```python
from build123d import *

# Parameters (mm, degrees)
BOSS_EXTRUDE1_DEPTH         = 50
BOSS_EXTRUDE2_START         = -50
BOSS_EXTRUDE2_DEPTH         = 50
TAP_DRILL_FOR_M5X0_8_TAP1_D = 4.2
CUT_EXTRUDE1_REACH          = 69.195
SKETCH5_W                   = 63.468496122
SKETCH5_H                   = 5.35


with BuildPart() as part:
    # Sketch1 → Boss-Extrude1 (new body)
    with BuildSketch(Plane.XY):
        with BuildLine():
            Line((-31.734248061, 1), (-17.721808598, 1))
            ThreePointArc((-17.721808598, 1), (0, 17.75), (17.721808598, 1))
            Line((17.721808598, 1), (31.734248061, 1))
            ThreePointArc((31.734248061, 1), (0, 31.75), (-31.734248061, 1))
        make_face()
    extrude(amount=BOSS_EXTRUDE1_DEPTH)

    # Sketch4 → Boss-Extrude2 (add)
    with BuildSketch(Plane.XY.offset(50).offset(BOSS_EXTRUDE2_START)):
        with BuildLine():
            Line((31.734248061, 31.75), (0, 31.75))
            ThreePointArc((0, 31.75), (22.094258304, 22.801452805), (31.734248061, 1))
            Line((31.734248061, 1), (31.734248061, 31.75))
        make_face()
        with BuildLine():
            ThreePointArc((-31.734248061, 1), (-22.094258304, 22.801452805), (0, 31.75))
            Line((0, 31.75), (-31.734248061, 31.75))
            Line((-31.734248061, 31.75), (-31.734248061, 1))
        make_face()
    extrude(amount=BOSS_EXTRUDE2_DEPTH)

    # Tap Drill for M5x0.8 Tap1 (through all)
    with Locations(Plane(origin=(-24.72802833, 1, 40), x_dir=(0, 0, -1), z_dir=(0, -1, 0))):
        with Locations((0, 0), (30, 0), (0, 49.45605666), (30, 49.45605666)):
            Hole(TAP_DRILL_FOR_M5X0_8_TAP1_D / 2)

    # Sketch5 → Cut-Extrude1 (cut, up to next)
    with BuildSketch(Plane.XY.offset(50), mode=Mode.PRIVATE) as cut_extrude1_sk1:
        with Locations((0, 29.075)):
            Rectangle(SKETCH5_W, SKETCH5_H)
    cut_extrude1_tool1 = extrude(cut_extrude1_sk1.sketch, amount=-CUT_EXTRUDE1_REACH, mode=Mode.PRIVATE) & part.part
    add(cut_extrude1_tool1.solids().sort_by_distance((0, 29.075, 50))[0], mode=Mode.SUBTRACT)


solid = part.part
```
Here's how the part is built. I have some questions about the finished solid (model axes, mm). Coordinates: 2 decimals unless noted, no trailing zeros. Loops run counter-clockwise (first coordinate to the right, second up) from the corner with the lowest first, then second, coordinate; pieces in that order, holes last. Notation, with made-up numbers: (7, 77) -> (57, 77) arc R29 cw to (57, 102) -> close; hole circle Ø2 at (88.5, -21). An arc over 180 degrees is marked (long way). Return JSON: item names as keys, results as strings.
1) Will this pin go through, and if not, where does the flat tip stop? pin 1 (2 mm diameter, centred on x = 0.5, z = 15, fed in from -Y).
Results below:
{"pin 1": "y = 17.69"}
2) If we section it at C-C, the plane x = 24: Write out the boundary of the cut face in (y, z), then the cut area to 3 significant figures.
Results below:
{"outline": "(1, 0) -> (26.4, 0) -> (26.4, 8.03) -> (1, 8.03) -> close; (1, 11.97) -> (26.4, 11.97) -> (26.4, 38.03) -> (1, 38.03) -> close; (1, 41.97) -> (26.4, 41.97) -> (26.4, 50) -> (1, 50) -> close", "area": "1,070 mm²"}
3) If we section it at A-A, the plane y = 4.5: Write out the boundary of the cut face in (x, z), then the cut area to 3 significant figures.
Results below:
{"outline": "(-31.73, 0) -> (-17.17, 0) -> (-17.17, 50) -> (-31.73, 50) -> close; (17.17, 0) -> (31.73, 0) -> (31.73, 50) -> (17.17, 50) -> close; hole circle Ø4.2 at (-24.73, 10); hole circle Ø4.2 at (-24.73, 40); hole circle Ø4.2 at (24.73, 10); hole circle Ø4.2 at (24.73, 40)", "area": "1,400 mm²"}
4) If we section it at B-B, the plane z = 10: Write out the boundary of the cut face in (x, y).
Results below:
{"outline": "(-31.73, 1) -> (-26.83, 1) -> (-26.83, 26.4) -> (-31.73, 26.4) -> close; (-22.63, 1) -> (-17.72, 1) arc R17.75 cw to (17.72, 1) -> (22.63, 1) -> (22.63, 26.4) -> (-22.63, 26.4) -> close; (26.83, 1) -> (31.73, 1) -> (31.73, 26.4) -> (26.83, 26.4) -> close"}
5) If we section it at D-D, the plane z = 16: Write out the boundary of the cut face in (x, y).
Results below:
{"outline": "(-31.73, 1) -> (-17.72, 1) arc R17.75 cw to (17.72, 1) -> (31.73, 1) -> (31.73, 26.4) -> (-31.73, 26.4) -> close"}
6) Thinking about a two-plate mould opening in Z: for faces 1 (the face through (26.147, 13.878, 38.452)), 2 (the face through (-25, 1, 25)), 3 (the face through (0, 20, 0)), which applies, +Z half, -Z half, draft (parallel to the pull), parting line (faces both ways), or undercut?
Results below:
{"face 1": "undercut", "face 2": "draft", "face 3": "-Z half"}
7) I need wall thicknesses on line 1 (X direction, y = 18.25, z = 40); line 2 (X direction, y = 11.25, z = 40); line 3 (X direction, y = 15.75, z = 10). Which ranges of each line are inside material? Lowest first, please. Write a range as from..to.
Results below:
{"line 1": "-31.73..-26.83, -22.63..22.63, 26.83..31.73", "line 2": "-31.73..-26.83, -22.63..-13.73, 13.73..22.63, 26.83..31.73", "line 3": "-31.73..-26.83, -22.63..-8.19, 8.19..22.63, 26.83..31.73"}
